Job drawing, mm, ordinate dimensions from the low corner. One solid piece. Give positions to 0.01 mm unless a question says otherwise; leave off trailing zeros. Order: outer loops, then holes, each group sorted by start corner. A loop starts at its lowest first (then second) coordinate and runs counter-clockwise, first axis right, second up. Notation, with made-up numbers: M 76.5,17 L 130.5,17 A32 ccw 130.5,43 Z; hole C 10,-40 d6. An arc over 180 degrees is marked long. Use CSV: the item, a comma, the result in double quotes. Start each with the question number.
Item 1: Band-saw the part on C-C on z = 34. Write the cut outline in (x, y) (1 decimal), plus the area to 3 significant figures.
Item 2: Band-saw the part on D-D on y = 4. Write the cut outline in (x, z) (1 decimal), plus the area to 3 significant figures.
Item 3: Band-saw the part on B-B on x = 2.35. Write the cut outline in (y, z), plus the area to 3 significant figures.
Item 4: Wall check: line 1 along Y through (x, z) = (1.1, 25.4); line 2 along Y through (x, z) = (2.05, 26.5); line 3 along Z through (x, y) = (2, 22.5) (1 decimal). Give the ranges that are in metal, low to high.
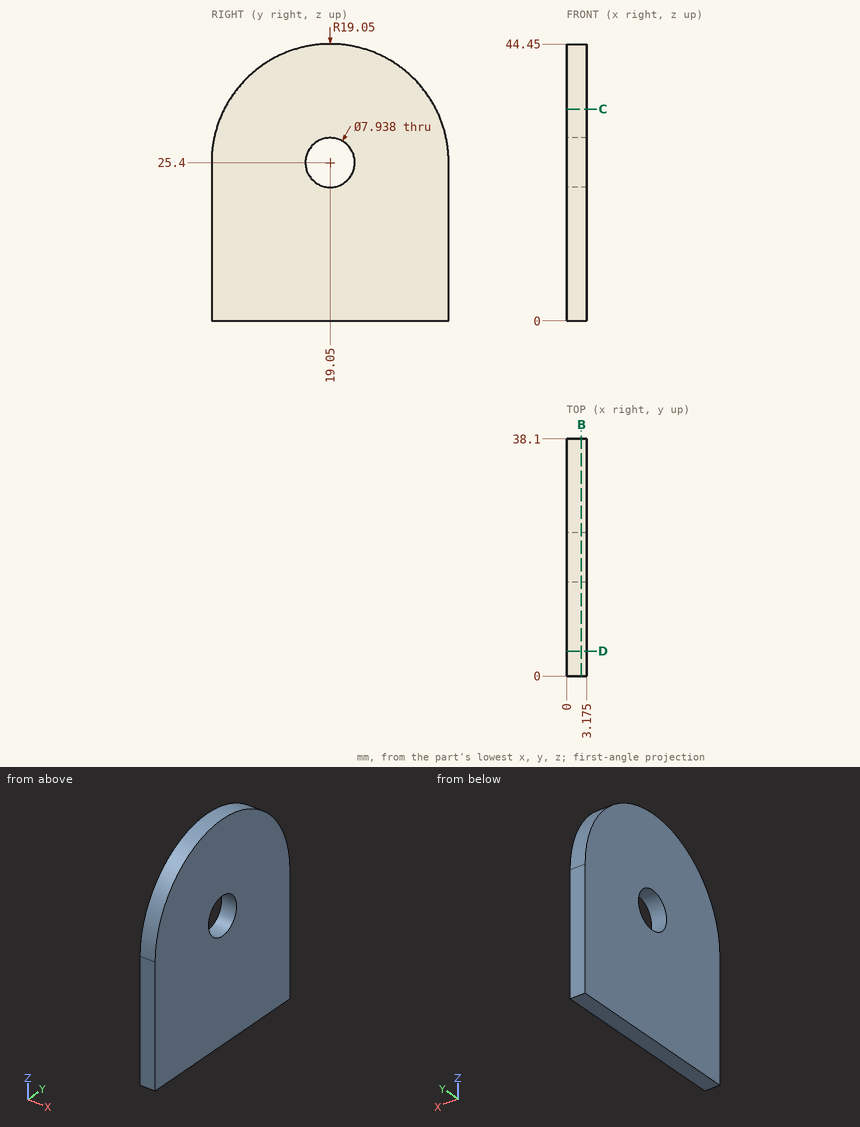
Model answer:
1,outline,"M 0,2.1 L 3.2,2.1 L 3.2,36 L 0,36 Z"
1,area,"108 mm^2"
2,outline,"M 0,0 L 3.2,0 L 3.2,37.1 L 0,37.1 Z"
2,area,"118 mm^2"
3,outline,"M 0,0 L 38.1,0 L 38.1,25.4 A19.05 ccw 0,25.4 Z; hole C 19.05,25.4 d7.94"
3,area,"1,490 mm^2"
4,line 1,"y = 0 to 15.08, 23.02 to 38.1"
4,line 2,"y = 0.03 to 15.24, 22.86 to 38.07"
4,line 3,"z = 0 to 23.4, 27.4 to 44.1"
